Autodesk Inventor part; units mm, degrees
ref_plane "YZ Plane" through (0, 0, 0) normal (1, 0, 0) x (0, 1, 0)
ref_plane "XZ Plane" through (0, 0, 0) normal (0, 1, 0) x (-1, 0, 0)
ref_plane "XY Plane" through (0, 0, 0) normal (0, 0, 1) x (1, 0, 0)
sketch "Sketch1" plane through (0, 0, 0) normal (0, 0, 1) x (1, 0, 0)
  circle A0 centre (0, 0) radius 18.2563
  dimension "d0" = 36.5125
extrude "Extrusion1" add sketch "Sketch1" along normal blind 228.6
chamfer "Chamfer1" distance 25.4 distance2 4.7625 1 edges at (-18.2563, 0, 228.6) measured on face at (18.1971, -1.469, 152.4)
chamfer "Chamfer2" distance 25.4 distance2 4.7625 1 edges at (-18.2563, 0, 0) measured on face at (18.0198, -2.9285, 135.4667)
properties part number "GE-12027-02"
CAD build for the part. Positions are in the model's coordinates, mm. Coordinates: 2 decimals unless noted, no trailing zeros. Order: outer loops, then holes, each group sorted by start corner. A loop starts at its lowest first (then second) coordinate and runs counter-clockwise, first axis right, second up. Notation, with made-up numbers: (83.5, -38) -> (125.5, -38) arc R28 cw to (125.5, -9) -> close; hole circle Ø1 at (-26, 8). An arc over 180 degrees is marked (long way). Answer in a Markdown table with one row per item.
1) Band-saw the part on D-D (z = 209). List the corners of the cut face in (x, y), and give its area (3 significant figures).
Check values:
| item | result |
|---|---|
| outline | circle Ø34.34 at (0, 0) |
| area | 926 mm2 |
2) Flat gauge pins, fed straight in: P1, Ø6, axis at y = -13, z = 42.5, coming from the +X side; P2, Ø5, axis at y = -7, z = 76, coming from the +X side; P3, Ø3, axis at x = -7, z = 129, coming from the -Y side. Where does each tip first touch, or does it go through?
Check values:
| item | result |
|---|---|
| P1 | x = 15.27 |
| P2 | x = 17.69 |
| P3 | y = -17.41 |
3) Band-saw the part on A-A (y = 0). List the corners of the cut face in (x, z).
Check values:
| item | result |
|---|---|
| outline | (-18.26, 25.4) -> (-13.49, 0) -> (13.49, 0) -> (18.26, 25.4) -> (18.26, 203.2) -> (13.49, 228.6) -> (-13.49, 228.6) -> (-18.26, 203.2) -> close |
4) Band-saw the part on C-C (z = 174). List the corners of the cut face in (x, y), and give its area (3 significant figures).
Check values:
| item | result |
|---|---|
| outline | circle Ø36.51 at (0, 0) |
| area | 1,050 mm2 |
5) Drill centre lines: line 1 (Y direction, x = 10.5, z = 162); line 2 (X direction, y = -14, z = 151); line 3 (X direction, y = 3, z = 26). Where is each one in solid material? Low to high.
Check values:
| item | result |
|---|---|
| line 1 | -14.93 to 14.93 |
| line 2 | -11.72 to 11.72 |
| line 3 | -18.01 to 18.01 |
